Geometry: see drawing. Coordinates: mm, zero at the bounding-box minimum. A direction names the side the tool comes from. Coordinates: 2 decimals unless noted, no trailing zeros. Loops run counter-clockwise (first coordinate to the right, second up) from the corner with the lowest first, then second, coordinate; pieces in that order, holes last. Notation, with made-up numbers: (89, 43) -> (142, 43) arc R31 cw to (142, 78) -> close; hole circle Ø10 at (-28.5, -29.5). An arc over 180 degrees is marked (long way). Put each result on its own line as item: value. Start each with the question number.
1) Contact query for flat-ended pins moving along their axis: P1, Ø2.5, axis at x = 18.66, z = 25.03, coming from the +Y side; P2, Ø2.5, axis at x = 4, y = 5, coming from the +Z side; P3, Ø15, axis at x = 19, y = 13.5, coming from the -Z side. Output: stop coordinate, or through.
2) Cut plane D-D (x = 2). Return the cut outline in (y, z), plus the area to 3 significant figures.
3) Cut plane C-C (z = 14). Return the cut outline in (x, y).
4) Cut plane B-B (y = 5). Return the cut outline in (x, z).
5) Cut plane A-A (x = 34). Return the cut outline in (y, z), plus the area to 3 significant figures.
6) Material intervals for L1, parallel to X at y = 28, z = 31; L2, parallel to Y at x = 34, z = 30.9; L3, parallel to Y at x = 22, z = 26.5, sorted ascending.
7) Set-up query: the marked faces 1 and 2. Return all of +Z, -Z, +X, -X, +Y, -Y with unobstructed straight access to the full face (end or side cutting, diameter ignored); none if empty.
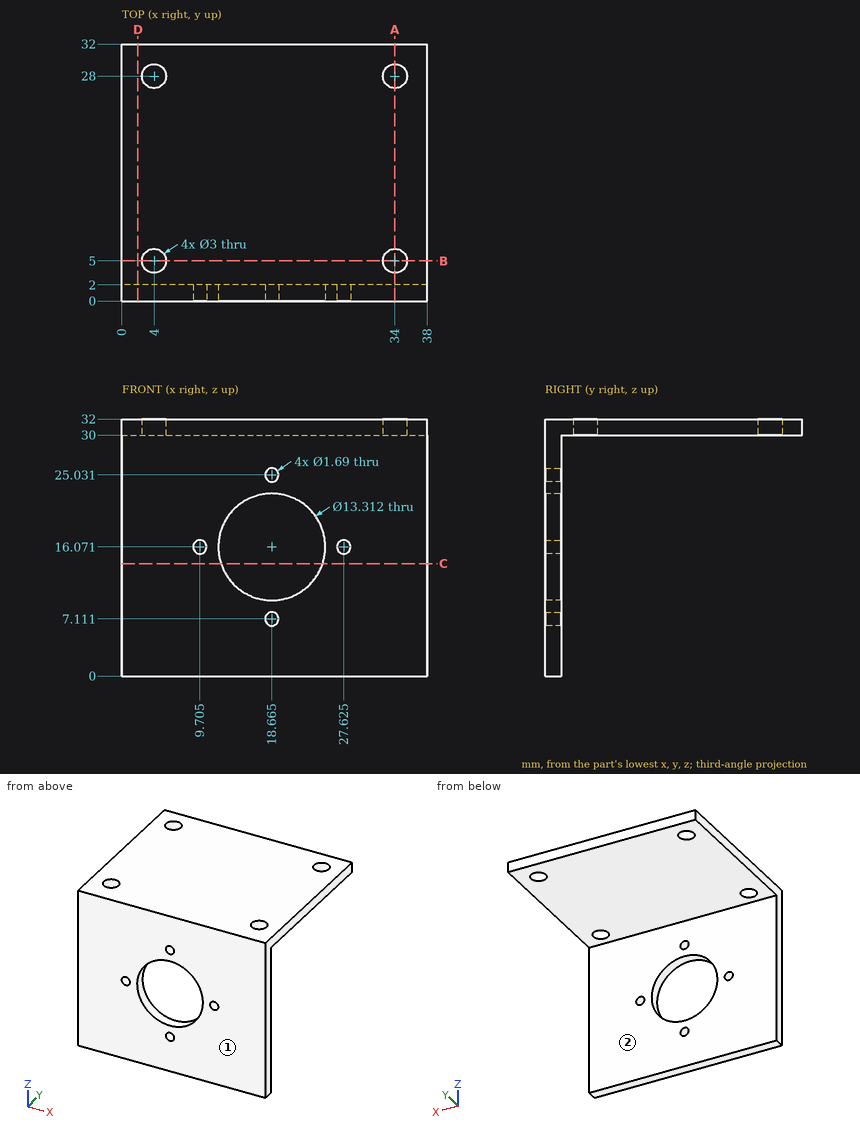
Results found:
1. P1: stops at y = 2
1. P2: passes through
1. P3: stops at z = 30
2. outline: (0, 0) -> (2, 0) -> (2, 30) -> (32, 30) -> (32, 32) -> (0, 32) -> close
2. area: 124 mm2
3. outline: (0, 0) -> (12.34, 0) -> (12.34, 2) -> (0, 2) -> close; (24.99, 0) -> (38, 0) -> (38, 2) -> (24.99, 2) -> close
4. outline: (0, 30) -> (2.5, 30) -> (2.5, 32) -> (0, 32) -> close; (5.5, 30) -> (32.5, 30) -> (32.5, 32) -> (5.5, 32) -> close; (35.5, 30) -> (38, 30) -> (38, 32) -> (35.5, 32) -> close
5. outline: (0, 0) -> (2, 0) -> (2, 30) -> (3.5, 30) -> (3.5, 32) -> (0, 32) -> close; (6.5, 30) -> (26.5, 30) -> (26.5, 32) -> (6.5, 32) -> close; (29.5, 30) -> (32, 30) -> (32, 32) -> (29.5, 32) -> close
5. area: 112 mm2
6. L1: x = 0 to 2.5, 5.5 to 32.5, 35.5 to 38
6. L2: y = 0 to 3.5, 6.5 to 26.5, 29.5 to 32
6. L3: y = 0 to 2
7. face 1: +Z, -Z, +X, -X, -Y
7. face 2: -Z, +X, -X, +Y
